Geometry: final body of the model. Coordinates: model frame, mm. Face numbers are marked on the shaded views. A direction names the side the tool comes from. Give positions to 0.01 mm unless a question says otherwise; leave off trailing zeros. Write each loop counter-clockwise with the first axis right and the second up, starting at its lowest first coordinate (ties: lowest second). Pieces come first, ordered by that corner, then holes.
Q1. Cut plane D-D on z = 4.75. Return the cut outline in (x, y), plus the area to 3 significant figures.
Q2. Cut plane B-B on y = -3.5. Return the cut outline in (x, z).
Q3. Line query: L1, parallel to Z at x = -10.32, y = -13.75; L2, parallel to X at y = -10.5, z = 3; L3, parallel to Y at x = 0.5, z = 10.5. Output: solid intervals per line, ascending.
Q4. Reachability of the marked faces 1, 2 and 3 from +Z, -Z, +X, -X, +Y, -Y: full face, straight path, thin tool, end or side. Return the list, or none.
Q5. Cut plane A-A on x = 17.8. Return the cut outline in (y, z).
Q6. Pin query (flat end, axial travel): pin 1 (5 mm diameter, centred on x = -18, z = 4.5, fed in from -Y); pin 2 (1.4 mm diameter, centred on x = 19.5, z = 7.5, fed in from -Y); pin 3 (3 mm diameter, centred on x = 16.5, z = 9, fed in from -Y). Return the tip coordinate at first contact, or that it passes through.
Q7. Cut plane C-C on x = -10.32. Return the cut outline in (y, z).
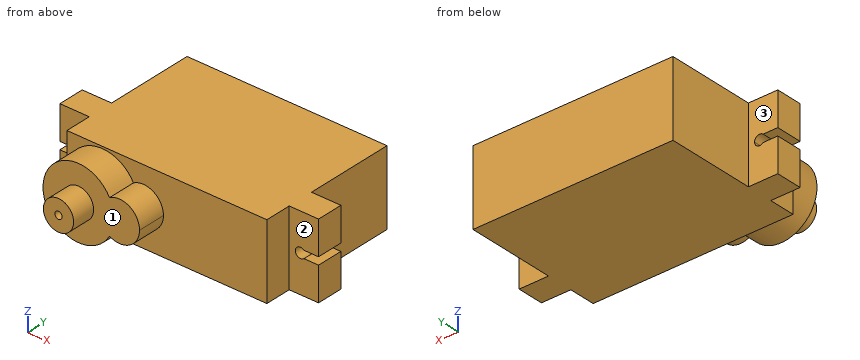
```python
from build123d import *

# Parameters (mm, degrees)
F0_W     = 32
F0_H     = 22.6
F1_DEPTH = 12
F3_START = -4.2
F3_DEPTH = 4.2
F4_R     = 2.42
F4_R_2   = 0.58
F5_DEPTH = 4.5
F6_R     = 2.42
F6_R_2   = 0.58
F7_DEPTH = 3.76


with BuildPart() as f1:
    # F0 (on Top) → F1 (new body)
    with BuildSketch(Plane.XY):
        Rectangle(F0_W, F0_H)
    extrude(amount=F1_DEPTH)

    # F2 (on face) → F3 (join)
    with BuildSketch(Plane.XZ.offset(11.3).offset(F3_START)):
        with BuildLine():
            Line((20.7, 12), (16, 12))
            Line((16, 12), (16, 0))
            Line((16, 0), (20.7, 0))
            Line((20.7, 0), (20.7, 5.4))
            Line((20.7, 5.4), (18.3589275445, 5.4))
            ThreePointArc((18.3589275445, 5.4), (16.98, 6), (18.3589275445, 6.6))
            Line((18.3589275445, 6.6), (20.7, 6.6))
            Line((20.7, 6.6), (20.7, 12))
        make_face()
        with BuildLine():
            Line((-16, 12), (-20.7, 12))
            Line((-20.7, 12), (-20.7, 6.6))
            Line((-20.7, 6.6), (-18.3589275445, 6.6))
            ThreePointArc((-18.3589275445, 6.6), (-17.4728307674, 6.7519044442), (-16.98, 6))
            ThreePointArc((-16.98, 6), (-17.4728307674, 5.2480955558), (-18.3589275445, 5.4))
            Line((-18.3589275445, 5.4), (-20.7, 5.4))
            Line((-20.7, 5.4), (-20.7, 0))
            Line((-20.7, 0), (-16, 0))
            Line((-16, 0), (-16, 12))
        make_face()
    extrude(amount=-F3_DEPTH)

    # F4 (on face) → F5 (join)
    with BuildSketch(Plane.XZ.offset(11.3)):
        with BuildLine():
            ThreePointArc((-5.3517097264, 3.2470939432), (-4.8208051156, 4.5782913016), (-4.64, 6))
            ThreePointArc((-4.64, 6), (-4.8208051156, 7.4217086984), (-5.3517097264, 8.7529060568))
            ThreePointArc((-5.3517097264, 8.7529060568), (-6.93, 6), (-5.3517097264, 3.2470939432))
        make_face()
        with BuildLine():
            ThreePointArc((-5.3517097264, 8.7529060568), (-4.8208051156, 7.4217086984), (-4.64, 6))
            ThreePointArc((-4.64, 6), (-4.8208051156, 4.5782913016), (-5.3517097264, 3.2470939432))
            ThreePointArc((-5.3517097264, 3.2470939432), (-2.1533768606, 3.2325594833), (-0.55, 6))
            ThreePointArc((-0.55, 6), (-2.1533768606, 8.7674405167), (-5.3517097264, 8.7529060568))
        make_face()
        with BuildLine():
            ThreePointArc((-5.3517097264, 3.2470939432), (-6.93, 6), (-5.3517097264, 8.7529060568))
            ThreePointArc((-5.3517097264, 8.7529060568), (-16, 6), (-5.3517097264, 3.2470939432))
        make_face()
        with Locations((-10.32, 6)):
            Circle(F4_R, mode=Mode.SUBTRACT)
        with Locations((-10.32, 6)):
            Circle(F4_R)
        with Locations((-10.32, 6)):
            Circle(F4_R_2, mode=Mode.SUBTRACT)
    extrude(amount=F5_DEPTH)

    # F6 (on face) → F7 (join)
    with BuildSketch(Plane.XZ.offset(15.8)):
        with Locations((-10.32, 6)):
            Circle(F6_R)
        with Locations((-10.32, 6)):
            Circle(F6_R_2, mode=Mode.SUBTRACT)
    extrude(amount=F7_DEPTH)


solid = f1.part
```
Data:
1. outline: (-20.7, -7.1) - (-16, -7.1) - (-16, -11.3) - (-15.86, -11.3) - (-15.86, -15.8) - (-12.39, -15.8) - (-12.39, -19.56) - (-8.25, -19.56) - (-8.25, -15.8) - (-0.81, -15.8) - (-0.81, -11.3) - (16, -11.3) - (16, -7.1) - (20.7, -7.1) - (20.7, -2.9) - (16, -2.9) - (16, 11.3) - (-16, 11.3) - (-16, -2.9) - (-20.7, -2.9) - close
1. area: 846 mm2
2. outline: (-20.7, 0) - (20.7, 0) - (20.7, 5.4) - (18.36, 5.4) arc R0.82 cw (long way) to (18.36, 6.6) - (20.7, 6.6) - (20.7, 12) - (-20.7, 12) - (-20.7, 6.6) - (-18.36, 6.6) arc R0.82 cw (long way) to (-18.36, 5.4) - (-20.7, 5.4) - close
3. L1: z = 0.32 to 5.42, 6.58 to 11.68
3. L2: x = -16 to 16
3. L3: y = -11.3 to 11.3
4. face 1: -Y
4. face 2: +Z, -Z, +X, -Y
4. face 3: +Z, -Z, -X, +Y
5. outline: (-7.1, 0) - (-2.9, 0) - (-2.9, 5.18) - (-7.1, 5.18) - close; (-7.1, 6.82) - (-2.9, 6.82) - (-2.9, 12) - (-7.1, 12) - close
6. pin 1: stops at y = -15.8
6. pin 2: stops at y = -7.1
6. pin 3: stops at y = -11.3
7. outline: (-19.56, 3.58) - (-15.8, 3.58) - (-15.8, 0.32) - (-11.3, 0.32) - (-11.3, 0) - (11.3, 0) - (11.3, 12) - (-11.3, 12) - (-11.3, 11.68) - (-15.8, 11.68) - (-15.8, 8.42) - (-19.56, 8.42) - (-19.56, 6.58) - (-11.3, 6.58) - (-11.3, 5.42) - (-19.56, 5.42) - close
